Geometry check sheet. Reference: the model listing, model coordinates, mm. A direction names the side the tool comes from. Round coordinates to 2 decimals unless told otherwise and drop trailing zeros. Loops run counter-clockwise (first coordinate to the right, second up) from the corner with the lowest first, then second, coordinate; pieces in that order, holes last. Notation, with made-up numbers: M 88.5,75.5 L 138.5,75.5 A21 ccw 138.5,96.5 Z; hole C 65,35 d7. An arc over 180 degrees is marked long. Write item = value, one per line.
from build123d import *

# Parameters (mm, degrees)
ESQUISSE1_W             = 310
ESQUISSE1_H             = 10
ESQUISSE1_W_2           = 10
ESQUISSE1_H_2           = 40
BOSS_EXTRU_1_DEPTH      = 200
ESQUISSE2_R             = 7.5
BOSS_EXTRU_2_DEPTH      = 20
ESQUISSE3_R             = 8
BOSS_EXTRU_3_DEPTH      = 200
ESQUISSE4_W             = 100
ESQUISSE4_H             = 45
ENL_V_MAT_EXTRU_1_DEPTH = 10


with BuildPart() as part:
    # Esquisse1 → Boss.-Extru.1 (new body)
    with BuildSketch(Plane.XY):
        with Locations((165, 5)):
            Rectangle(ESQUISSE1_W, ESQUISSE1_H)
        with Locations((5, 30)):
            Rectangle(ESQUISSE1_W_2, ESQUISSE1_H_2)
        with Locations((5, 5)):
            Rectangle(ESQUISSE1_W_2, ESQUISSE1_H)
    extrude(amount=BOSS_EXTRU_1_DEPTH)

    # Esquisse2 → Boss.-Extru.2 (add)
    with BuildSketch(Plane(origin=(0, 10, 0), x_dir=(1, 0, 0), z_dir=(0, 1, 0))):
        with Locations(Location((90, -25, 0), (0, 0, 270))):
            Circle(ESQUISSE2_R)
        with Locations(Location((90, -175, 0), (0, 0, 270))):
            Circle(ESQUISSE2_R)
    extrude(amount=BOSS_EXTRU_2_DEPTH)

    # Esquisse3 → Boss.-Extru.3 (add)
    with BuildSketch(Plane(origin=(0, 10, 0), x_dir=(1, 0, 0), z_dir=(0, 1, 0))):
        with Locations(Location((260, -20, 0), (0, 0, 270))):
            Circle(ESQUISSE3_R)
        with Locations(Location((260, -180, 0), (0, 0, 270))):
            Circle(ESQUISSE3_R)
    extrude(amount=-BOSS_EXTRU_3_DEPTH)

    # Esquisse4 → Enlèv. mat.-Extru.1 (cut)
    with BuildSketch(Plane(origin=(0, 10, 0), x_dir=(1, 0, 0), z_dir=(0, 1, 0))):
        with Locations((270, -100)):
            Rectangle(ESQUISSE4_W, ESQUISSE4_H)
    extrude(amount=-ENL_V_MAT_EXTRU_1_DEPTH, mode=Mode.SUBTRACT)


solid = part.part
(1) Material ranges on line 1 along Y through (x, z) = (236, 45); line 2 along Z through (x, y) = (295, 4); line 3 along X through (y, z) = (25, 178), recorded low to high. Write a range as from..to.
Result set:
line_1 = 0..10
line_2 = 0..77.5, 122.5..200
line_3 = 0..10, 83.13..96.87
(2) Sectioned sample at B-B on z = 159. Record the cut outline in (x, y), then the cut area to 3 significant figures.
Result set:
outline = M 0,0 L 320,0 L 320,10 L 10,10 L 10,50 L 0,50 Z
area = 3,600 mm2
(3) Tool access check on faces 1 (the flat face through (136, 7, 200)), 2 (the flat face through (90, 30, 25)), 3 (the cylindrical face through (267.932, -93.67, 18.959)), 4 (the flat face through (5, 50, 99)), 5 (the flat face through (269, 5, 122.5)). Record the directions out of +Z, -Z, +X, -X, +Y, -Y that give a thin tool (end or side, any length) a straight path to the whole face; none if there is none.
Result set:
face_1 = +Z, +X, -X, +Y, -Y
face_2 = +Z, -Z, +X, +Y
face_3 = -Y
face_4 = +Z, -Z, +X, -X, +Y
face_5 = +X, +Y, -Y
(4) Sectioned sample at C-C on y = -12.5. Record the cut outline in (x, z).
Result set:
outline = C 260,20 d16; C 260,180 d16
(5) Sectioned sample at A-A on x = 236.5. Record the cut outline in (y, z), then the cut area to 3 significant figures.
Result set:
outline = M 0,0 L 10,0 L 10,77.5 L 0,77.5 Z; M 0,122.5 L 10,122.5 L 10,200 L 0,200 Z
area = 1,550 mm2
(6) Sectioned sample at D-D on x = 90. Record the cut outline in (y, z).
Result set:
outline = M 0,0 L 10,0 L 10,17.5 L 30,17.5 L 30,32.5 L 10,32.5 L 10,167.5 L 30,167.5 L 30,182.5 L 10,182.5 L 10,200 L 0,200 Z
(7) Release check for a two-part mould opening along X. For faces 6 (the flat face through (320, 5, 38)), 7 (the flat face through (260, -190, 20)), 8 (the cylindrical face through (87.13, 19.86, 181.93)), 9 (the cylindrical face through (82.68, 19.86, 23.37)) record: released by +X, released by -X, zero draft, split by the parting line, or undercut.
Result set:
face_6 = released by +X
face_7 = zero draft
face_8 = undercut
face_9 = undercut
(8) Depth check by flat-ended pin: pin 1 Ø10 at (y, z) = (-55.5, 165.5) entering from -X; pin 2 Ø16.5 at (x, z) = (90, 23.5) entering from +Y; pin 3 Ø2 at (x, z) = (34.5, 51) entering from +Y; pin 4 Ø3 at (x, z) = (104, 147.5) entering from -Y. Enter the tip coordinate at first touch or a pass-through.
Result set:
pin_1 = through
pin_2 = 30
pin_3 = 10
pin_4 = 0
